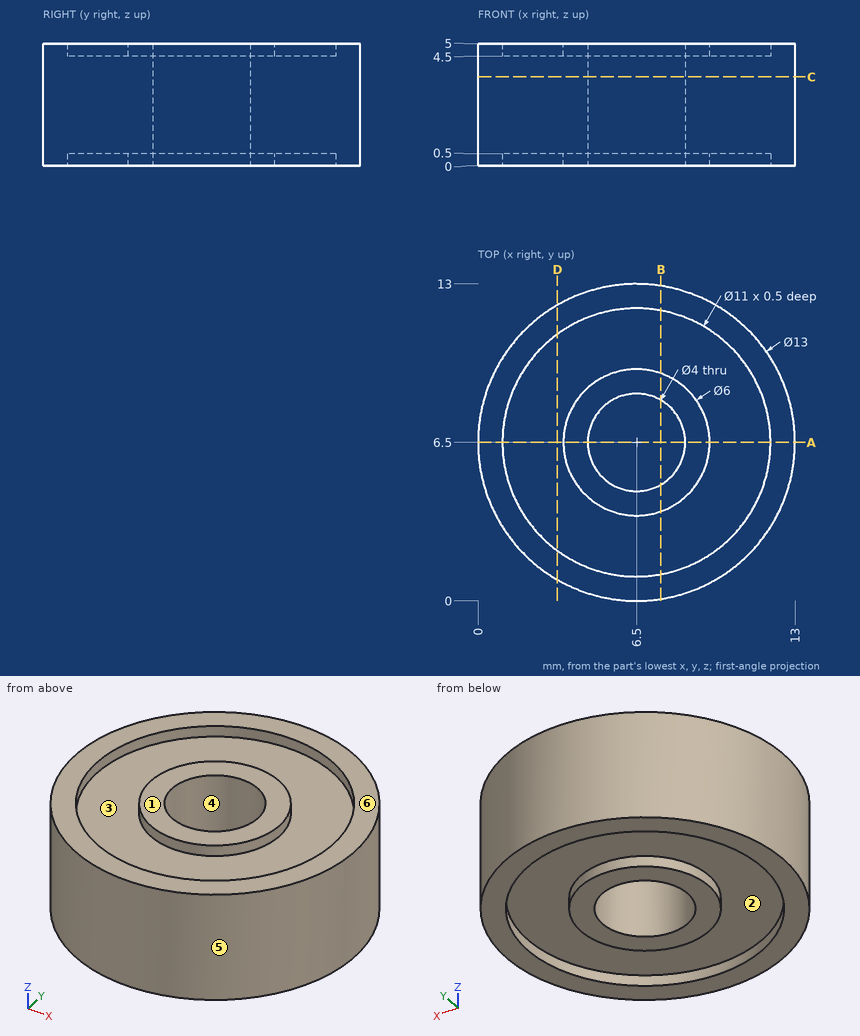
Can you work these out from the drawing? Everything is in mm from the part's minimum corner. A direction names the side the tool comes from. Round coordinates to 2 decimals unless told otherwise and drop trailing zeros. Write each loop counter-clockwise with the first axis right and the second up, starting at its lowest first coordinate (ties: lowest second). Pieces come first, ordered by that corner, then holes. Notation, with made-up numbers: (14, -9) - (66, -9) arc R23 ccw to (66, 8) - close; hole circle Ø10 at (67, 19.25). An arc over 180 degrees is marked (long way). Write each question's results on one line, items separated by ' | '. Start each with the question number.
1) Suppose I cut it at B-B (x = 7.5). List the corners of the cut face in (y, z) for me, and give its area (3 significant figures).
2) Suppose I cut it at A-A (y = 6.5). List the corners of the cut face in (x, z) for me, and give its area (3 significant figures).
3) Suppose I cut it at C-C (z = 3.65). List the corners of the cut face in (x, y) for me, and give its area (3 significant figures).
4) We'd pull the mould along Y, two halves only. Please class the marked faces 4, 5 and 6: released by +Y, released by -Y, zero draft, split by the parting line, or undercut.
5) For pin 1 Ø1.5 at (x, z) = (8, 3) entering from +Y; pin 2 Ø1.5 at (x, z) = (2, 2) entering from +Y; pin 3 Ø1.5 at (x, z) = (8.5, 1) entering from -Y, each with a flat end and sliding along its axis, tell me the tip position at first contact or that it passes through.
6) Which directions (+Z, -Z, +X, -X, +Y, -Y) give clear straight access to the entire face, cutting with the end or side of a thin tool? Please do the marked faces 1, 2 and 3.
7) Suppose I cut it at D-D (x = 3.25). List the corners of the cut face in (y, z) for me, and give its area (3 significant figures).
8) Please list where these lines run through material, in increasing order: line 1 (Y direction, x = 6.5, z = 4.85); line 2 (Y direction, x = 6.5, z = 1.85); line 3 (X direction, y = 6, z = 0.75).
Here are the results:
1) outline: (0.08, 0) - (1.09, 0) - (1.09, 0.5) - (3.67, 0.5) - (3.67, 0) - (4.77, 0) - (4.77, 5) - (3.67, 5) - (3.67, 4.5) - (1.09, 4.5) - (1.09, 5) - (0.08, 5) - close; (8.23, 0) - (9.33, 0) - (9.33, 0.5) - (11.91, 0.5) - (11.91, 0) - (12.92, 0) - (12.92, 5) - (11.91, 5) - (11.91, 4.5) - (9.33, 4.5) - (9.33, 5) - (8.23, 5) - close | area: 41.7 mm2
2) outline: (0, 0) - (1, 0) - (1, 0.5) - (3.5, 0.5) - (3.5, 0) - (4.5, 0) - (4.5, 5) - (3.5, 5) - (3.5, 4.5) - (1, 4.5) - (1, 5) - (0, 5) - close; (8.5, 0) - (9.5, 0) - (9.5, 0.5) - (12, 0.5) - (12, 0) - (13, 0) - (13, 5) - (12, 5) - (12, 4.5) - (9.5, 4.5) - (9.5, 5) - (8.5, 5) - close | area: 40.0 mm2
3) outline: circle Ø13 at (6.5, 6.5); hole circle Ø4 at (6.5, 6.5) | area: 120 mm2
4) face 4: undercut | face 5: split by the parting line | face 6: zero draft
5) pin 1: stops at y = 12.96 | pin 2: stops at y = 11.81 | pin 3: stops at y = 0.12
6) face 1: +Z, +X, -X, +Y, -Y | face 2: -Z | face 3: +Z
7) outline: (0.87, 0) - (2.06, 0) - (2.06, 0.5) - (10.94, 0.5) - (10.94, 0) - (12.13, 0) - (12.13, 5) - (10.94, 5) - (10.94, 4.5) - (2.06, 4.5) - (2.06, 5) - (0.87, 5) - close | area: 47.4 mm2
8) line 1: y = 0 to 1, 3.5 to 4.5, 8.5 to 9.5, 12 to 13 | line 2: y = 0 to 4.5, 8.5 to 13 | line 3: x = 0.02 to 4.56, 8.44 to 12.98
